Geometry: final body of the model. Coordinates: model frame, mm. A direction names the side the tool comes from. Coordinates: 2 decimals unless noted, no trailing zeros. Loops run counter-clockwise (first coordinate to the right, second up) from the corner with the lowest first, then second, coordinate; pieces in that order, holes last. Notation, with made-up numbers: (76, 76.5) -> (85, 76.5) arc R20 ccw to (85, 86.5) -> close; hole circle Ø2 at (-23, -37). An arc over 180 degrees is marked (long way). One line per item, written item: value. Start each with the question number.
Item 1: Section query A-A on z = 31.5. Return loops of the section in (x, y).
Item 2: Ray query, probe 1 along X at (y, z) = (73.5, 11.5); probe 2 along X at (y, z) = (36, 24.5); probe 3 along Y at (x, z) = (-9.5, 15.5). Return the intervals inside material, ascending. Write a range as from..to.
Item 3: Section query C-C on y = -19.5. Return loops of the section in (x, z), then the cut area to 3 significant figures.
Item 4: Contact query for a flat-ended pin moving along its axis: pin 1 Ø3 at (x, y) = (39, 18.5) entering from +Z. Output: stop coordinate, or through.
Item 5: Mould query, pull axis X, two halves, no side actions, for faces 4 (the flat face through (-70, 1, 40)), 5 (the flat face through (-1, 1, 10)), 6 (the flat face through (-75, -1, 20)). Classes: +X half, -X half, draft (parallel to the pull), parting line (faces both ways), or undercut.
Item 6: Section query B-B on x = -30. Return loops of the section in (y, z).
Item 7: Section query D-D on x = 40.5. Return loops of the section in (y, z).
Item 8: Set-up query: faces 1 (the flat face through (55, 75, 25)), 2 (the flat face through (-1, -80, 20)), 3 (the flat face through (-60, 70, 25)). Return all of +Z, -Z, +X, -X, +Y, -Y with unobstructed straight access to the full face (end or side cutting, diameter ignored); none if empty.
from build123d import *

# Parameters (mm, degrees)
F0_W      = 150
F0_H      = 160
F1_DEPTH  = 10
F2_W      = 150
F2_H      = 160
F2_W_2    = 130
F2_H_2    = 140
F3_DEPTH  = 30
F4_W      = 20
F4_H      = 10
F5_DEPTH  = 30
F6_W      = 30
F6_H      = 10
F7_DEPTH  = 30
F8_W      = 20
F8_H      = 10
F9_DEPTH  = 30
F10_W     = 30
F10_H     = 10
F11_DEPTH = 30


with BuildPart() as f1:
    # F0 (on Top) → F1 (new body)
    with BuildSketch(Plane.XY):
        Rectangle(F0_W, F0_H)
    extrude(amount=F1_DEPTH)

    # F2 (on face) → F3 (join)
    with BuildSketch(Plane.XY.offset(10)):
        Rectangle(F2_W, F2_H)
        Rectangle(F2_W_2, F2_H_2, mode=Mode.SUBTRACT)
    extrude(amount=F3_DEPTH)

    # F4 (on face) → F5 (cut)
    with BuildSketch(Plane.XY.offset(40)):
        with Locations((-45, 75)):
            Rectangle(F4_W, F4_H)
    extrude(amount=-F5_DEPTH, mode=Mode.SUBTRACT)

    # F6 (on face) → F7 (cut)
    with BuildSketch(Plane.XY.offset(40)):
        with Locations((40, 75)):
            Rectangle(F6_W, F6_H)
    extrude(amount=-F7_DEPTH, mode=Mode.SUBTRACT)

    # F8 (on face) → F9 (cut)
    with BuildSketch(Plane.XY.offset(40)):
        with Locations((-45, -75)):
            Rectangle(F8_W, F8_H)
    extrude(amount=-F9_DEPTH, mode=Mode.SUBTRACT)

    # F10 (on face) → F11 (cut)
    with BuildSketch(Plane.XY.offset(40)):
        with Locations((40, -75)):
            Rectangle(F10_W, F10_H)
    extrude(amount=-F11_DEPTH, mode=Mode.SUBTRACT)


solid = f1.part
Reply:
1. outline: (-75, -80) -> (-55, -80) -> (-55, -70) -> (-65, -70) -> (-65, 70) -> (-55, 70) -> (-55, 80) -> (-75, 80) -> close; (-35, -80) -> (25, -80) -> (25, -70) -> (-35, -70) -> close; (-35, 70) -> (25, 70) -> (25, 80) -> (-35, 80) -> close; (55, -80) -> (75, -80) -> (75, 80) -> (55, 80) -> (55, 70) -> (65, 70) -> (65, -70) -> (55, -70) -> close
2. probe 1: x = -75..-55, -35..25, 55..75
2. probe 2: x = -75..-65, 65..75
2. probe 3: y = -80..-70, 70..80
3. outline: (-75, 0) -> (75, 0) -> (75, 40) -> (65, 40) -> (65, 10) -> (-65, 10) -> (-65, 40) -> (-75, 40) -> close
3. area: 2,100 mm²
4. pin 1: stops at z = 10
5. face 4: draft
5. face 5: undercut
5. face 6: -X half
6. outline: (-80, 0) -> (80, 0) -> (80, 40) -> (70, 40) -> (70, 10) -> (-70, 10) -> (-70, 40) -> (-80, 40) -> close
7. outline: (-80, 0) -> (80, 0) -> (80, 10) -> (-80, 10) -> close
8. face 1: +Z, +Y, -Y
8. face 2: +Z, -Z, +X, -X, -Y
8. face 3: +Z
